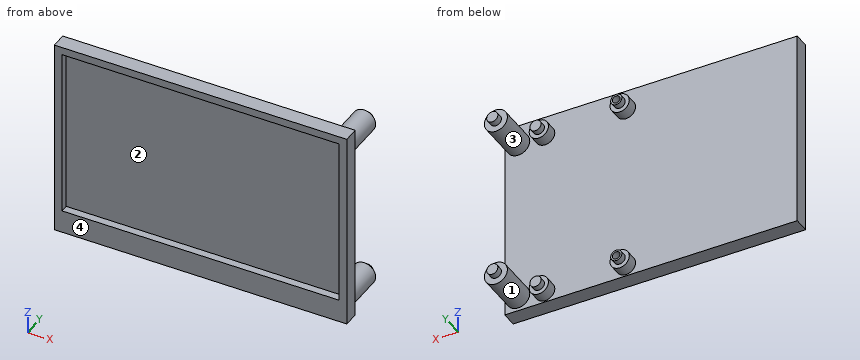
```python
from build123d import *

# Parameters (mm, degrees)
SKETCH1_W           = 76
SKETCH1_H           = 48
SKETCH1_W_2         = 72
SKETCH1_H_2         = 44
BOSS_EXTRUDE1_DEPTH = 2
SKETCH2_W           = 76
SKETCH2_H           = 48
BOSS_EXTRUDE2_DEPTH = 2
SKETCH8_W           = 76
SKETCH8_H           = 4
BOSS_EXTRUDE7_DEPTH = 4
SKETCH3_R           = 2.5
SKETCH3_R_2         = 1
BOSS_EXTRUDE3_DEPTH = 3
SKETCH4_R           = 1.45
SKETCH4_R_2         = 1
BOSS_EXTRUDE4_DEPTH = 1.6
SKETCH5_R           = 3
BOSS_EXTRUDE5_DEPTH = 10.6
SKETCH7_R           = 1.45
BOSS_EXTRUDE6_DEPTH = 1.7


with BuildPart() as part:
    # Sketch1 → Boss-Extrude1 (new body)
    with BuildSketch(Plane(origin=(0, 0, 0), x_dir=(1, 0, 0), z_dir=(0, 1, 0))):
        with Locations((36, 22)):
            Rectangle(SKETCH1_W, SKETCH1_H)
        with Locations((36, 22)):
            Rectangle(SKETCH1_W_2, SKETCH1_H_2, mode=Mode.SUBTRACT)
    extrude(amount=BOSS_EXTRUDE1_DEPTH)

    # Sketch2 → Boss-Extrude2 (add)
    with BuildSketch(Plane(origin=(0, 2, 0), x_dir=(1, 0, 0), z_dir=(0, 1, 0))):
        with Locations((36, 22)):
            Rectangle(SKETCH2_W, SKETCH2_H)
    extrude(amount=BOSS_EXTRUDE2_DEPTH)

    # Sketch8 → Boss-Extrude7 (add)
    with BuildSketch(Plane(origin=(0, 0, -46), x_dir=(-1, 0, 0), z_dir=(0, 0, -1))):
        with Locations((-36, 2)):
            Rectangle(SKETCH8_W, SKETCH8_H)
    extrude(amount=BOSS_EXTRUDE7_DEPTH)

    # Sketch3 → Boss-Extrude3 (add)
    # profile 1 of 4: a face of its own
    with BuildSketch(Plane(origin=(0, 4, 0), x_dir=(1, 0, 0), z_dir=(0, 1, 0))):
        with Locations(Location((42.5, 3.25, 0), (0, 0, 90))):
            Circle(SKETCH3_R)
        with Locations(Location((42.5, 3.25, 0), (0, 0, 270))):
            Circle(SKETCH3_R_2, mode=Mode.SUBTRACT)
    # profile 2 of 4: a face of its own
    with BuildSketch(Plane(origin=(0, 4, 0), x_dir=(1, 0, 0), z_dir=(0, 1, 0))):
        with Locations(Location((63.5, 3.25, 0), (0, 0, 90))):
            Circle(SKETCH3_R)
    # profile 3 of 4: a face of its own
    with BuildSketch(Plane(origin=(0, 4, 0), x_dir=(1, 0, 0), z_dir=(0, 1, 0))):
        with Locations(Location((42.5, 47.15, 0), (0, 0, 90))):
            Circle(SKETCH3_R)
        with Locations(Location((42.5, 47.15, 0), (0, 0, 270))):
            Circle(SKETCH3_R_2, mode=Mode.SUBTRACT)
    # profile 4 of 4: a face of its own
    with BuildSketch(Plane(origin=(0, 4, 0), x_dir=(1, 0, 0), z_dir=(0, 1, 0))):
        with Locations(Location((63.5, 47.15, 0), (0, 0, 90))):
            Circle(SKETCH3_R)
    extrude(amount=BOSS_EXTRUDE3_DEPTH)

    # Sketch4 → Boss-Extrude4 (add)
    # profile 1 of 4: a face of its own
    with BuildSketch(Plane(origin=(0, 7, 0), x_dir=(1, 0, 0), z_dir=(0, 1, 0))):
        with Locations(Location((42.5, 3.25, 0), (0, 0, 270))):
            Circle(SKETCH4_R)
        with Locations(Location((42.5, 3.25, 0), (0, 0, 270))):
            Circle(SKETCH4_R_2, mode=Mode.SUBTRACT)
    # profile 2 of 4: a face of its own
    with BuildSketch(Plane(origin=(0, 7, 0), x_dir=(1, 0, 0), z_dir=(0, 1, 0))):
        with Locations(Location((42.5, 47.15, 0), (0, 0, 270))):
            Circle(SKETCH4_R)
        with Locations(Location((42.5, 47.15, 0), (0, 0, 270))):
            Circle(SKETCH4_R_2, mode=Mode.SUBTRACT)
    # profile 3 of 4: a face of its own
    with BuildSketch(Plane(origin=(0, 7, 0), x_dir=(1, 0, 0), z_dir=(0, 1, 0))):
        with Locations(Location((63.5, 3.25, 0), (0, 0, 270))):
            Circle(SKETCH4_R)
    # profile 4 of 4: a face of its own
    with BuildSketch(Plane(origin=(0, 7, 0), x_dir=(1, 0, 0), z_dir=(0, 1, 0))):
        with Locations(Location((63.5, 47.15, 0), (0, 0, 270))):
            Circle(SKETCH4_R)
    extrude(amount=BOSS_EXTRUDE4_DEPTH)

    # Sketch5 → Boss-Extrude5 (add)
    with BuildSketch(Plane(origin=(0, 4, 0), x_dir=(1, 0, 0), z_dir=(0, 1, 0))):
        with Locations(Location((70.5, 3.25, 0), (0, 0, 90))):
            Circle(SKETCH5_R)
        with Locations(Location((70.5, 46.25, 0), (0, 0, 90))):
            Circle(SKETCH5_R)
    extrude(amount=BOSS_EXTRUDE5_DEPTH)

    # Sketch7 → Boss-Extrude6 (add)
    with BuildSketch(Plane(origin=(0, 14.6, 0), x_dir=(1, 0, 0), z_dir=(0, 1, 0))):
        with Locations(Location((70.5, 3.25, 0), (0, 0, 270))):
            Circle(SKETCH7_R)
        with Locations(Location((70.5, 46.15, 0), (0, 0, 270))):
            Circle(SKETCH7_R)
    extrude(amount=BOSS_EXTRUDE6_DEPTH)


solid = part.part
```
The listing builds one solid part. Answer for the finished solid, in the listing's coordinates (mm). Face numbers are marked on the shaded views. A direction names the side the tool comes from. Round coordinates to 2 decimals unless told otherwise and drop trailing zeros. Loops run counter-clockwise (first coordinate to the right, second up) from the corner with the lowest first, then second, coordinate; pieces in that order, holes last.
Q1. Section B-B, the plane z = -11.5 is taken. Determine the outline of the cut face in (x, y), then the cut area to 3 significant figures.
Q2. Which of the six approach directions +Z, -Z, +X, -X, +Y, -Y give full straight-line access (tool end or side, diameter ignored) to the marked faces 1 and 2?
Q3. Section A-A, the plane x = 63.5 is taken. Determine the outline of the cut face in (y, z).
Q4. Find the intervals of material crossed by line 1 (X direction, y = 6.5, z = -3.25); line 2 (X direction, y = 1.25, z = -41.5); line 3 (Z direction, x = 14.5, y = 1.75), in increasing order.
Q5. Section C-C, the plane y = 13.75 is taken. Determine the outline of the cut face in (x, z).
Q6. Given pin 1 Ø2.5 at (x, z) = (64, -4) entering from +Y; pin 2 Ø13 at (x, z) = (47, -18) entering from -Y; pin 3 Ø1.5 at (x, z) = (13, -42) entering from +Y; pin 4 Ø3 at (x, z) = (42.5, -47.15) entering from -Y, each flat-ended and moving along its own axis, determine where each tip first touches the part or whether it passes through.
Q7. For a pull along Z with two mould halves and no side action, classify the marked faces 3 and 4 as released by +Z, released by -Z, zero draft, split by the parting line, or undercut.
Completed:
1. outline: (-2, 0) - (0, 0) - (0, 2) - (72, 2) - (72, 0) - (74, 0) - (74, 4) - (-2, 4) - close
1. area: 160 mm2
2. face 1: +Y
2. face 2: -Y
3. outline: (0, -50) - (4, -50) - (4, -49.65) - (7, -49.65) - (7, -48.6) - (8.6, -48.6) - (8.6, -45.7) - (7, -45.7) - (7, -44.65) - (4, -44.65) - (4, -5.75) - (7, -5.75) - (7, -4.7) - (8.6, -4.7) - (8.6, -1.8) - (7, -1.8) - (7, -0.75) - (4, -0.75) - (4, 2) - (0, 2) - (0, 0) - (2, 0) - (2, -44) - (0, -44) - close
4. line 1: x = 40 to 41.5, 43.5 to 45, 61 to 66, 67.5 to 73.5
4. line 2: x = -2 to 0, 72 to 74
4. line 3: z = -50 to -44, 0 to 2
5. outline: circle Ø6 at (70.5, -46.25); circle Ø6 at (70.5, -3.25)
6. pin 1: stops at y = 8.6
6. pin 2: stops at y = 2
6. pin 3: stops at y = 4
6. pin 4: stops at y = 0
7. face 3: undercut
7. face 4: zero draft
